For this review, use the dimensioned drawing (mm, ordinates from the lowest corner) and the shaded views. Coordinates: 2 decimals unless noted, no trailing zeros. Write each loop counter-clockwise with the first axis right and the second up, starting at its lowest first coordinate (ties: lowest second). Pieces come first, ordered by that corner, then holes. Notation, with made-up numbers: (3, 21.25) - (23, 21.25) arc R22 ccw to (23, 36.25) - close; hole circle Ø10 at (28.25, -18.75). An arc over 180 degrees is marked (long way). Use one line per item in the form item = value. Start each with the question number.
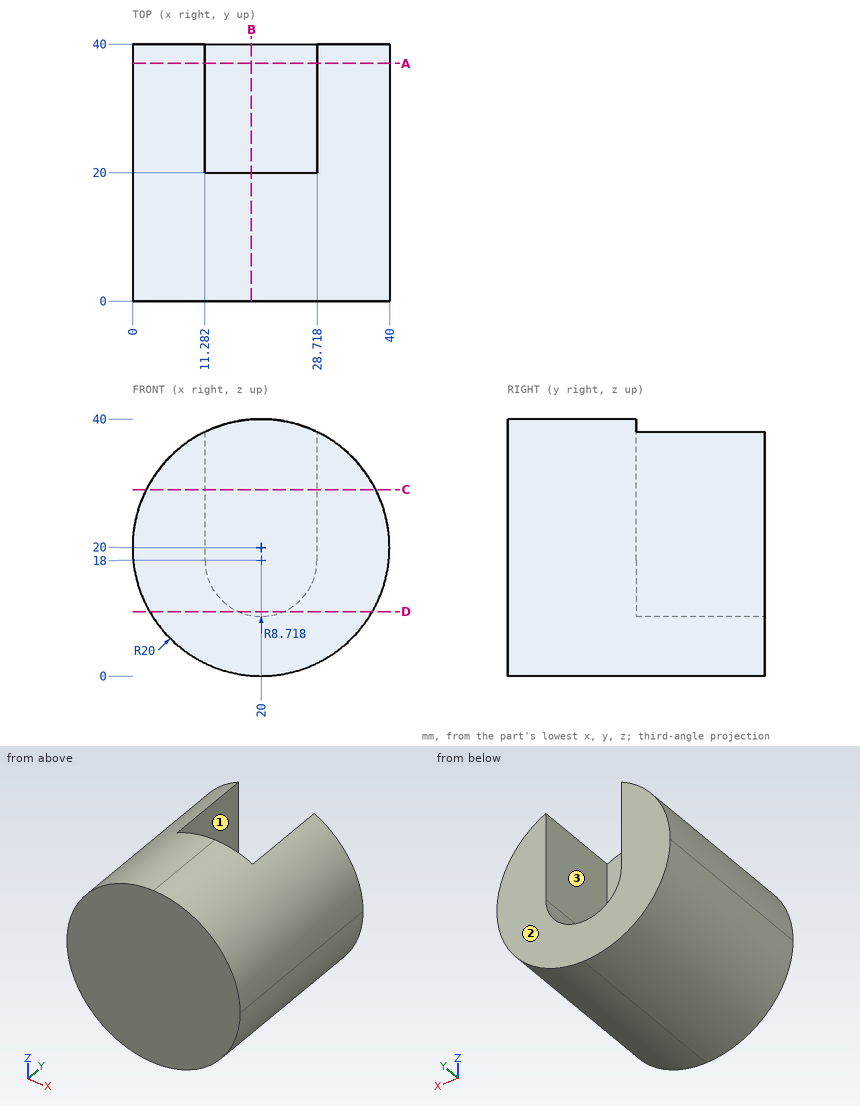
1. Take a section at A-A (y = 37). State the section outline as (x, z) points.
2. Take a section at B-B (x = 18.5). State the section outline as (y, z) points.
3. Take a section at C-C (z = 29). State the section outline as (x, y) points.
4. Take a section at D-D (z = 10). State the section outline as (x, y) points.
5. The part is to be moulded in two halves that separate along X. For the marked faces 1, 2 and 3, say which applies: released by +X, released by -X, zero draft, split by the parting line, or undercut.
6. For P1, Ø1, axis at x = 8.5, y = 34.5, coming from the +Z side; P2, Ø1.5, axis at y = 15.5, z = 26.5, coming from the -X side; P3, Ø10, axis at y = 27, z = 27.5, coming from the -X side, all flat-tipped, find the tip position at first contact; note any pin that passes through.
7. For L1, parallel to X at y = 26.5, z = 25.5; L2, parallel to Y at x = 26.5, z = 33; L3, parallel to X at y = 32, z = 18, list the stretches that pass through material, from the lowest coordinate up.
Returned:
q1.outline = (11.28, 18) - (11.28, 38) arc R20 ccw (long way) to (28.72, 38) - (28.72, 18) arc R8.72 cw to start
q2.outline = (0, 0.06) - (40, 0.06) - (40, 9.41) - (20, 9.41) - (20, 39.94) - (0, 39.94) - close
q3.outline = (2.14, 0) - (37.86, 0) - (37.86, 40) - (28.72, 40) - (28.72, 20) - (11.28, 20) - (11.28, 40) - (2.14, 40) - close
q4.outline = (2.68, 0) - (37.32, 0) - (37.32, 40) - (23.46, 40) - (23.46, 20) - (16.54, 20) - (16.54, 40) - (2.68, 40) - close
q5.face_1 = undercut
q5.face_2 = zero draft
q5.face_3 = undercut
q6.P1 = 36.7
q6.P2 = 0.84
q6.P3 = 0.16
q7.L1 = 0.77 to 11.28, 28.72 to 39.23
q7.L2 = 0 to 20
q7.L3 = 0.1 to 11.28, 28.72 to 39.9
